Job drawing, mm, ordinate dimensions from the low corner. One solid piece. A direction names the side the tool comes from. Round coordinates to 2 decimals unless told otherwise and drop trailing zeros. Write each loop counter-clockwise with the first axis right and the second up, starting at its lowest first coordinate (ties: lowest second). Pieces come first, ordered by that corner, then holes. Notation, with made-up numbers: M 31.5,-14 L 37.5,-14 A24 ccw 37.5,21 Z; hole C -4.75,86 d9. An arc over 180 degrees is marked long. Answer as a JSON object with one key per item and string values. Group by question number.
1. Band-saw the part on A-A, the plane x = 19.05. Write the cut outline in (y, z) (3 decimals), plus the area to 3 significant figures.
2. Drill centre line: line 1 (Z direction, x = 15, y = 20). Where is it in solid material? Low to high. Write a range as from..to.
3. Drop a flat-ended pin along its axis: pin 1 (8 mm diameter, centred on x = 11.5, y = 4, fed in from +Z). Give the stop position or say it passes through.
4. Band-saw the part on D-D, the plane x = 4.5. Write the cut outline in (y, z), plus the area to 3 significant figures.
5. Band-saw the part on C-C, the plane z = 52. Write the cut outline in (x, y) (3 decimals).
6. Which spindle directions (+Z, -Z, +X, -X, +Y, -Y) get a long thin tool onto all of the face, cutting with end or side? Do the marked faces 1 and 2. Say none if no direction does.
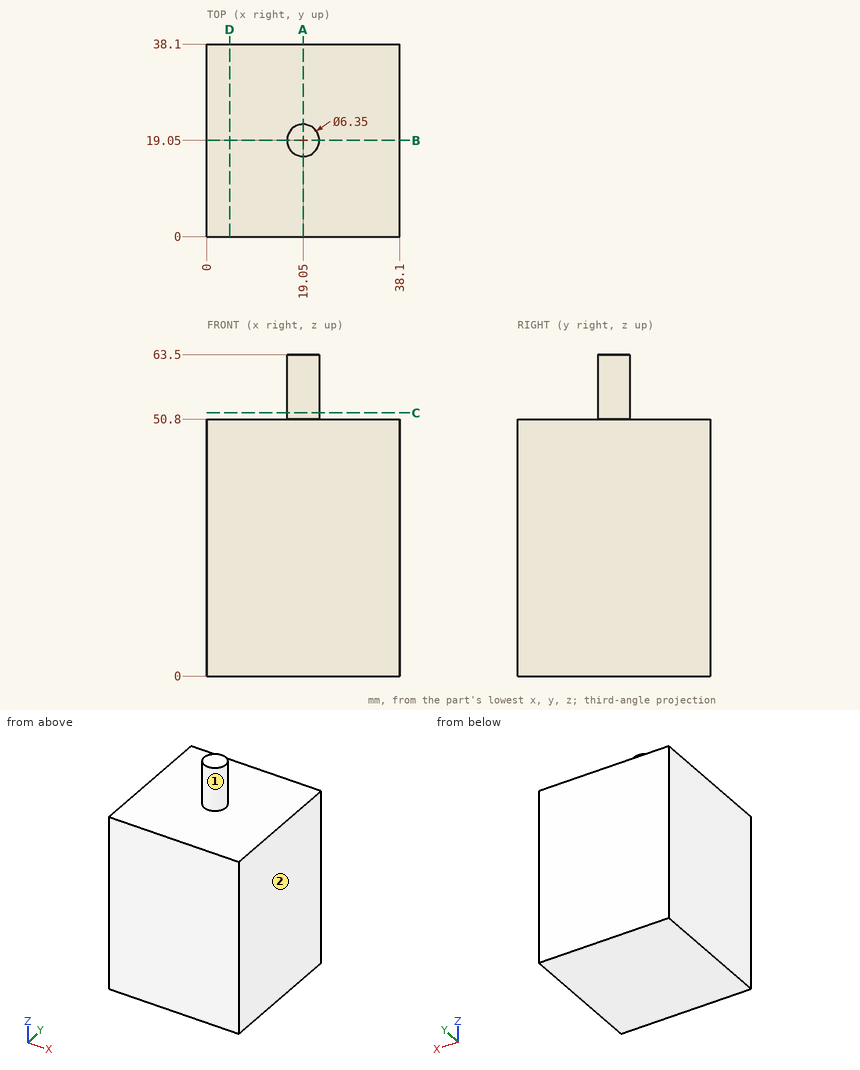
Worked answers:
{
 "1": {"outline": "M 0,0 L 38.1,0 L 38.1,50.8 L 22.225,50.8 L 22.225,63.5 L 15.875,63.5 L 15.875,50.8 L 0,50.8 Z", "area": "2,020 mm^2"},
 "2": {"line 1": "z = 0..50.8"},
 "3": {"pin 1": "stops at z = 50.8"},
 "4": {"outline": "M 0,0 L 38.1,0 L 38.1,50.8 L 0,50.8 Z", "area": "1,940 mm^2"},
 "5": {"outline": "C 19.05,19.05 d6.35"},
 "6": {"face 1": "+Z", "face 2": "+Z, -Z, +X, +Y, -Y"}
}
